Answer from the drawing. Dimensions are ordinates in mm from the lowest x, y and z of the part. A direction names the side the tool comes from. Coordinates: 2 decimals unless noted, no trailing zeros. Order: outer loops, then holes, each group sorted by start corner. A loop starts at its lowest first (then second) coordinate and runs counter-clockwise, first axis right, second up. Notation, with made-up numbers: (-34.75, 44.5) -> (-18.75, 44.5) arc R21 ccw to (-18.75, 49.5) -> close; hole circle Ø3 at (78, -20.75). An arc over 180 degrees is marked (long way). Answer as a JSON object with one key per item and string values. Group by question number.
1) Section A-A on y = 44.5 is taken. Determine the outline of the cut face in (x, z), and give its area (3 significant figures).
2) Consider L1, parallel to Y at x = 17.5, z = 0.95; L2, parallel to X at y = 19, z = 4.85; L3, parallel to Y at x = 8, z = 1.9. Determine where each line is inside the solid, lowest interval first.
3) A tool of negligible diameter and unlimited length cuts with its end or side. For the marked faces 1, 2 and 3, from which of +Z, -Z, +X, -X, +Y, -Y can it reach the whole face along a straight path? Write none if from no direction.
4) Given pin 1 (0.6 mm diameter, centred on x = 5, z = 1, fed in from +Y); pin 2 (5.5 mm diameter, centred on x = 17.5, y = 3.5, fed in from +Z); pin 3 (1.2 mm diameter, centred on x = 19.5, z = 4.5, fed in from +Y); pin 4 (1.5 mm diameter, centred on y = 8, z = 3, fed in from -X), each flat-ended and moving along its own axis, determine where each tip first touches the part or whether it passes through.
5) Section B-B on z = 5.35 is taken. Determine the outline of the cut face in (x, y), and give its area (3 significant figures).
6) Section C-C on x = 13 is taken. Determine the outline of the cut face in (y, z), and give its area (3 significant figures).
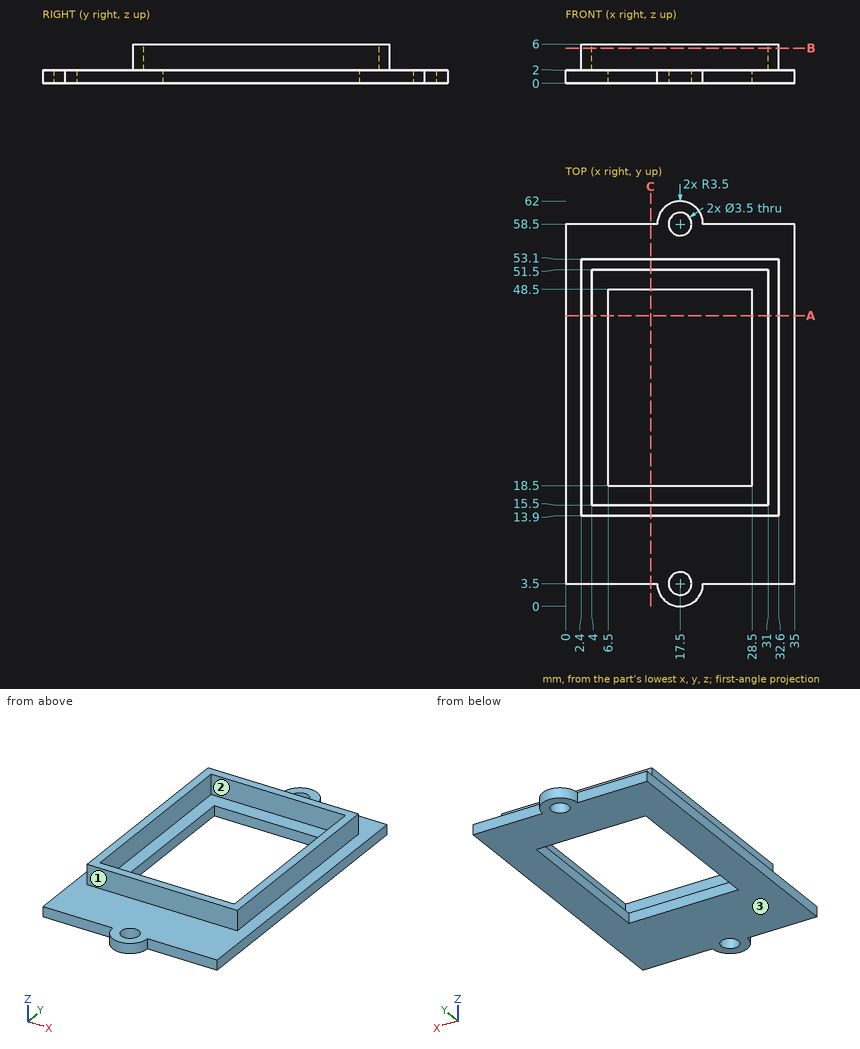
Worked answers:
{
 "1": {"outline": "(0, 0) -> (6.5, 0) -> (6.5, 2) -> (4, 2) -> (4, 6) -> (2.4, 6) -> (2.4, 2) -> (0, 2) -> close; (28.5, 0) -> (35, 0) -> (35, 2) -> (32.6, 2) -> (32.6, 6) -> (31, 6) -> (31, 2) -> (28.5, 2) -> close", "area": "38.8 mm²"},
 "2": {"L1": "y = 0 to 1.75, 5.25 to 18.5, 48.5 to 56.75, 60.25 to 62", "L2": "x = 2.4 to 4, 31 to 32.6", "L3": "y = 3.5 to 18.5, 48.5 to 58.5"},
 "3": {"face 1": "+Z, +X, -X, -Y", "face 2": "+Z", "face 3": "-Z, +X, -X, +Y, -Y"},
 "4": {"pin 1": "stops at y = 58.5", "pin 2": "stops at z = 2", "pin 3": "stops at y = 53.1", "pin 4": "passes through"},
 "5": {"outline": "(2.4, 13.9) -> (32.6, 13.9) -> (32.6, 53.1) -> (2.4, 53.1) -> close; hole (4, 15.5) -> (31, 15.5) -> (31, 51.5) -> (4, 51.5) -> close", "area": "212 mm²"},
 "6": {"outline": "(3.5, 0) -> (18.5, 0) -> (18.5, 2) -> (15.5, 2) -> (15.5, 6) -> (13.9, 6) -> (13.9, 2) -> (3.5, 2) -> close; (48.5, 0) -> (58.5, 0) -> (58.5, 2) -> (53.1, 2) -> (53.1, 6) -> (51.5, 6) -> (51.5, 2) -> (48.5, 2) -> close", "area": "62.8 mm²"}
}
